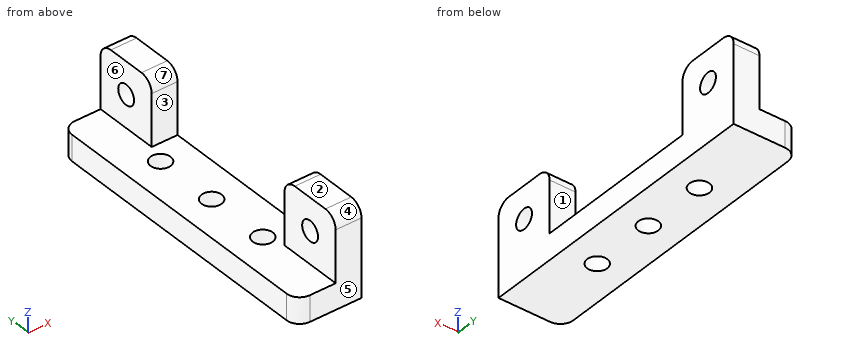
from build123d import *

# Parameters (mm, degrees)
SKETCH1_W           = 10
SKETCH1_H           = 46
SKETCH1_R           = 1.55
BOSS_EXTRUDE1_DEPTH = 4
SKETCH2_W           = 4
SKETCH2_H           = 10
BOSS_EXTRUDE2_DEPTH = 10
CUT_EXTRUDE1_REACH  = 6
SKETCH3_R           = 1.55
FILLET1_R           = 2


with BuildPart() as part:
    # Sketch1 → Boss-Extrude1 (new body)
    with BuildSketch(Plane.XY):
        Rectangle(SKETCH1_W, SKETCH1_H)
        with Locations((0, 10)):
            Circle(SKETCH1_R, mode=Mode.SUBTRACT)
        Circle(SKETCH1_R, mode=Mode.SUBTRACT)
        with Locations((0, -10)):
            Circle(SKETCH1_R, mode=Mode.SUBTRACT)
    extrude(amount=BOSS_EXTRUDE1_DEPTH)

    # Sketch2 → Boss-Extrude2 (add)
    with BuildSketch(Plane.XY.offset(4)):
        with Locations((3, 18)):
            Rectangle(SKETCH2_W, SKETCH2_H)
        with Locations((3, -18)):
            Rectangle(SKETCH2_W, SKETCH2_H)
    extrude(amount=BOSS_EXTRUDE2_DEPTH)

    # Sketch3 → Cut-Extrude1 (cut, up to next)
    with BuildSketch(Plane.ZY.offset(-1), mode=Mode.PRIVATE) as cut_extrude1_sk1:
        with Locations((9, 18)):
            Circle(SKETCH3_R)
    cut_extrude1_tool1 = extrude(cut_extrude1_sk1.sketch, amount=-CUT_EXTRUDE1_REACH, mode=Mode.PRIVATE) & part.part
    add(cut_extrude1_tool1.solids().sort_by_distance((1, 18, 9))[0], mode=Mode.SUBTRACT)
    # Sketch3 → Cut-Extrude1 (cut, up to next)
    with BuildSketch(Plane.ZY.offset(-1), mode=Mode.PRIVATE) as cut_extrude1_sk2:
        with Locations((9, -18)):
            Circle(SKETCH3_R)
    cut_extrude1_tool2 = extrude(cut_extrude1_sk2.sketch, amount=-CUT_EXTRUDE1_REACH, mode=Mode.PRIVATE) & part.part
    add(cut_extrude1_tool2.solids().sort_by_distance((1, -18, 9))[0], mode=Mode.SUBTRACT)

    # Fillet1
    fillet1_edges = [part.edges().sort_by_distance(p)[0] for p in [
        (3, 23, 14),
        (3, 13, 14),
        (3, -13, 14),
        (3, -23, 14),
        (-5, -23, 2),
        (-5, 23, 2),
    ]]
    fillet(fillet1_edges, radius=FILLET1_R)


solid = part.part
Read the model definition and answer for the solid it produces. Units are mm, in the model's axes. Face numbers are marked on the shaded views. A direction names the side the tool comes from. Coordinates: 2 decimals unless noted, no trailing zeros. Loops run counter-clockwise (first coordinate to the right, second up) from the corner with the lowest first, then second, coordinate; pieces in that order, holes last. Notation, with made-up numbers: (14.25, 2) -> (60.25, 2) arc R20 cw to (60.25, 22) -> close; hole circle Ø1 at (44, 57.5). An arc over 180 degrees is marked (long way). Write item = value, one per line. Start each with the question number.
1) The part is cut by section B-B, the plane z = 1. Determine the outline of the cut face in (x, y).
2) The part is cut by section A-A, the plane y = -18. Determine the outline of the cut face in (x, z).
3) For the marked faces 5, 6 and 7, determine the directions among +Z, -Z, +X, -X, +Y, -Y from which every point of the face is accessible in a straight line to the end or side of a thin tool.
4) The mould has two halves that part along Y. Classify the marked faces 1, 2, 3 and 4: pulls with the +Y half, pulls with the -Y half, needs draft (parallel to the pull), parting line crosses it, or undercut.
5) The part is cut by section D-D, the plane x = 4. Determine the outline of the cut face in (y, z), plus the area to 3 significant figures.
6) The part is cut by section C-C, the plane x = 0. Determine the outline of the cut face in (y, z).
7) Given P1, Ø3, axis at y = -17.5, z = 7, coming from the -X side; P2, Ø3, axis at x = 0, y = 0, coming from the +Z side; P3, Ø1.5, axis at x = -3.5, y = 1, coming from the +Z side, each flat-ended and moving along its own axis, determine where each tip first touches the part or whether it passes through.
8) Find the intervals of material crossed by L1, parallel to Y at x = 0, z = 2.2; L2, parallel to Y at x = 3.6, z = 9; L3, parallel to Z at x = 0.25, y = 14, in increasing order. Write a range as from..to.
Result:
q1.outline = (-5, -21) arc R2 ccw to (-3, -23) -> (5, -23) -> (5, 23) -> (-3, 23) arc R2 ccw to (-5, 21) -> close; hole circle Ø3.1 at (0, -10); hole circle Ø3.1 at (0, 0); hole circle Ø3.1 at (0, 10)
q2.outline = (-5, 0) -> (5, 0) -> (5, 7.45) -> (1, 7.45) -> (1, 4) -> (-5, 4) -> close; (1, 10.55) -> (5, 10.55) -> (5, 14) -> (1, 14) -> close
q3.face_5 = +Z, -Z, +X, -X, -Y
q3.face_6 = +Z, -X, +Y, -Y
q3.face_7 = +Z, +X, -X
q4.face_1 = undercut
q4.face_2 = needs draft
q4.face_3 = undercut
q4.face_4 = pulls with the -Y half
q5.outline = (-23, 0) -> (23, 0) -> (23, 12) arc R2 ccw to (21, 14) -> (15, 14) arc R2 ccw to (13, 12) -> (13, 4) -> (-13, 4) -> (-13, 12) arc R2 ccw to (-15, 14) -> (-21, 14) arc R2 ccw to (-23, 12) -> close; hole circle Ø3.1 at (-18, 9); hole circle Ø3.1 at (18, 9)
q5.area = 365 mm²
q6.outline = (-23, 0) -> (-11.55, 0) -> (-11.55, 4) -> (-23, 4) -> close; (-8.45, 0) -> (-1.55, 0) -> (-1.55, 4) -> (-8.45, 4) -> close; (1.55, 0) -> (8.45, 0) -> (8.45, 4) -> (1.55, 4) -> close; (11.55, 0) -> (23, 0) -> (23, 4) -> (11.55, 4) -> close
q7.P1 = 1
q7.P2 = through
q7.P3 = 4
q8.L1 = -23..-11.55, -8.45..-1.55, 1.55..8.45, 11.55..23
q8.L2 = -23..-19.55, -16.45..-13, 13..16.45, 19.55..23
q8.L3 = 0..4
